Autodesk Inventor part; units mm, degrees
ref_plane "YZ Plane" through (0, 0, 0) normal (1, 0, 0) x (0, 1, 0)
ref_plane "XZ Plane" through (0, 0, 0) normal (0, 1, 0) x (-1, 0, 0)
ref_plane "XY Plane" through (0, 0, 0) normal (0, 0, 1) x (1, 0, 0)
sketch "Sketch1" plane through (0, 0, 0) normal (1, 0, 0) x (0, 1, 0)
  line L0 (4.45, 9.25) -> (4.45, -9.25)
  line L1 (4.45, -9.25) -> (-1.8065, -9.25)
  arc A0 (-1.8065, -9.25) -> (-4.45, 7.7812) centre (-6.45, -1.25) ccw
  line L2 (4.45, 9.25) -> (-4.45, 9.25)
  circle A1 centre (-6.45, -1.25) radius 9.15 construction
  line L3 (4.45, 6.063) -> (-0.7859, 6.063) construction
  line L4 (-4.45, 9.25) -> (-4.45, 7.7812)
  point P0 (0, 0)
  point P1 (0, 9.25)
  point P2 (4.45, 0)
  dimension "d0" = 10.9
  dimension "d1" = 18.3
  dimension "d2" = 0.1
  dimension "d6" = 8
  dimension "d7" = 7.313
  dimension "d9" = 2
  dimension "d19" = 10.5
extrude "Extrusion1" add sketch "Sketch1" along normal mid plane 10.4
sketch "Sketch2" plane through (-5.2, 4.45, 9.25) normal (0, 1, 0) x (1, 0, 0)
  line L0 (0, 0) -> (10.4, 0)
  line L1 (10.4, 18.5) -> (10.4, 0)
  line L2 (10.4, 18.5) -> (0, 18.5)
  line L3 (0, 0) -> (0, 18.5)
  line L4 (0, 0) -> (10.4, 0) construction
  line L5 (5.2, 0) -> (5.2, 18.5) construction
  line L6 (10.4, 18.5) -> (0, 18.5) construction
  point P0 (5.2, 9.25)
  point P1 (5.2, 3.187)
  point P2 (5.2, 3.187)
  point P3 (5.2, 3.187)
  point P4 (5.2, 3.187)
hole "Hole1" at (0, 4.45, 6.063) at (0, 4.45, 6.063) direction (0, -1, 0) diameter 2.459 end through all
fillet "Fillet1" radius 1 2 edges at (0, 4.45, 9.25) (0, 4.45, -9.25)
fillet "Fillet1" radius 0.5 2 edges at (0, -4.45, 9.25) (0, -4.45, 7.7812)
fillet "Fillet1" radius 0.25 1 edges at (0, -1.8065, -9.25)
chamfer "Chamfer1" distance 0.25 angle 45 20 edges at (5.2, -0.25, 9.25) (5.2, -4.3036, 9.1036) (5.2, -4.45, 8.462) (5.2, -4.3463, 7.8692) (5.2, 2.6527, 0.3942) (5.2, -1.1939, -9.0759) (5.2, 1.2472, -9.25) (5.2, 4.1571, -8.9571) (5.2, 4.45, 0) (5.2, 4.1571, 8.9571) (-5.2, -0.25, 9.25) (-5.2, 4.1571, 8.9571) (-5.2, 4.45, 0) (-5.2, 4.1571, -8.9571) (-5.2, 1.2472, -9.25) (-5.2, -1.1939, -9.0759) (-5.2, 2.6527, 0.3942) (-5.2, -4.3463, 7.8692) (-5.2, -4.45, 8.462) (-5.2, -4.3036, 9.1036)
properties part number "EPS_BatteryHeatsink" material "Aluminum 6061"
The model under review builds one solid part; all positions refer to its coordinate system, in mm. Round coordinates to 2 decimals unless told otherwise and drop trailing zeros. Loops run counter-clockwise (first coordinate to the right, second up) from the corner with the lowest first, then second, coordinate; pieces in that order, holes last. Notation, with made-up numbers: (37, 41.5) -> (95, 41.5) arc R24 cw to (95, 79.5) -> close; hole circle Ø4 at (79, -28.75). An arc over 180 degrees is marked (long way). One line per question, with ' | ' between items. Start each with the question number.
Item 1: Draft analysis for pull direction Z (two halves, no side actions). For faces 1 (the face through (-5.074, 4.077, 8.863)), 2 (the face through (-0.069, 2.625, 0.538)), 3 (the face through (-0.069, 4.165, -8.949)), state which applies: +Z half, -Z half, draft (parallel to the pull), parting line (faces both ways), or undercut.
Item 2: Add section C-C, the plane y = 1.75. Count the separate pieces of the cut face and the enclosed holes in it, then the cut area to 3 significant figures.
Item 3: For pin 1 (6 mm diameter, centred on x = 3, z = -4, fed in from -Y); pin 2 (5 mm diameter, centred on x = -3, z = -3.5, fed in from -Y), all flat-tipped, find the tip position at first contact; note any pin that passes through.
Item 4: Wall thickness on line 1 along Z through (x, y) = (-2.75, 0.5); line 2 along X through (y, z) = (2, 5.75); line 3 along Y through (x, z) = (4.5, -1.5): over which ranges is each line inside the solid? List them lowest first. Write a range as [from, to].
Item 5: Add section A-A, the plane x = 0. Write out the cut boundary in (y, z), then the cut area to 3 significant figures.
Item 6: Add section B-B, the plane x = -3.75. Write out the cut boundary in (y, z).
Return value:
1) face 1: +Z half | face 2: undercut | face 3: -Z half
2) separate pieces: 2 | enclosed holes: 1 | area: 98.2 mm2
3) pin 1: stops at y = 0.8 | pin 2: stops at y = 1.49
4) line 1: z = [-9.25, -7.35], [4.85, 9.25] | line 2: x = [-5.2, -1.19], [1.19, 5.2] | line 3: y = [2.8, 4.45]
5) outline: (-4.45, 8.17) arc R0.5 ccw to (-4.08, 7.69) arc R9.25 cw to (-2.9, 7.29) -> (4.45, 7.29) -> (4.45, 8.25) arc R1 ccw to (3.45, 9.25) -> (-3.95, 9.25) arc R0.5 ccw to (-4.45, 8.75) -> close; (-1.1, -8.8) arc R0.25 ccw to (-0.96, -9.25) -> (3.45, -9.25) arc R1 ccw to (4.45, -8.25) -> (4.45, 4.83) -> (0.52, 4.83) arc R9.25 cw to start | area: 54.7 mm2
6) outline: (-4.45, 8.17) arc R0.5 ccw to (-4.08, 7.69) arc R9.25 cw to (-1.1, -8.8) arc R0.25 ccw to (-0.96, -9.25) -> (3.45, -9.25) arc R1 ccw to (4.45, -8.25) -> (4.45, 8.25) arc R1 ccw to (3.45, 9.25) -> (-3.95, 9.25) arc R0.5 ccw to (-4.45, 8.75) -> close
